The drawing under review shows one solid part. Ordinate dimensions are in mm from its lowest x, y, z. Coordinates: 2 decimals unless noted, no trailing zeros. Loops run counter-clockwise (first coordinate to the right, second up) from the corner with the lowest first, then second, coordinate; pieces in that order, holes last. Notation, with made-up numbers: (27, 86.5) - (71, 86.5) arc R9 ccw to (71, 99.5) - close; hole circle Ø10 at (-8.75, 89.25). An arc over 180 degrees is marked (long way). Answer as a JSON object with one key per item and string values. Group by question number.
Item 1: Clearance check with flat-ended pins moving along their axes: pin 1 (1.5 mm diameter, centred on x = 20.5, y = 2, fed in from +Z); pin 2 (1.5 mm diameter, centred on x = 60, y = 1, fed in from +Z). State where each tip first meets the part, or that it passes through.
Item 2: To check wall thickness, follow line 1 (Z direction, x = 17.5, y = 1.8); line 2 (X direction, y = 2.55, z = 16) (1 decimal); line 3 (X direction, y = 1.5, z = 35.5). State the ranges of each line that lie inside material, in increasing order.
Item 3: We need section B-B (x = 53.5). Give the boundary of the cut face in (y, z), then the cut area to 3 significant figures.
Item 4: We need section C-C (z = 7). Give the boundary of the cut face in (x, y).
Item 5: We need section A-A (z = 18). Give the boundary of the cut face in (x, y).
Item 6: We need section D-D (y = 1.2). Give the boundary of the cut face in (x, z).
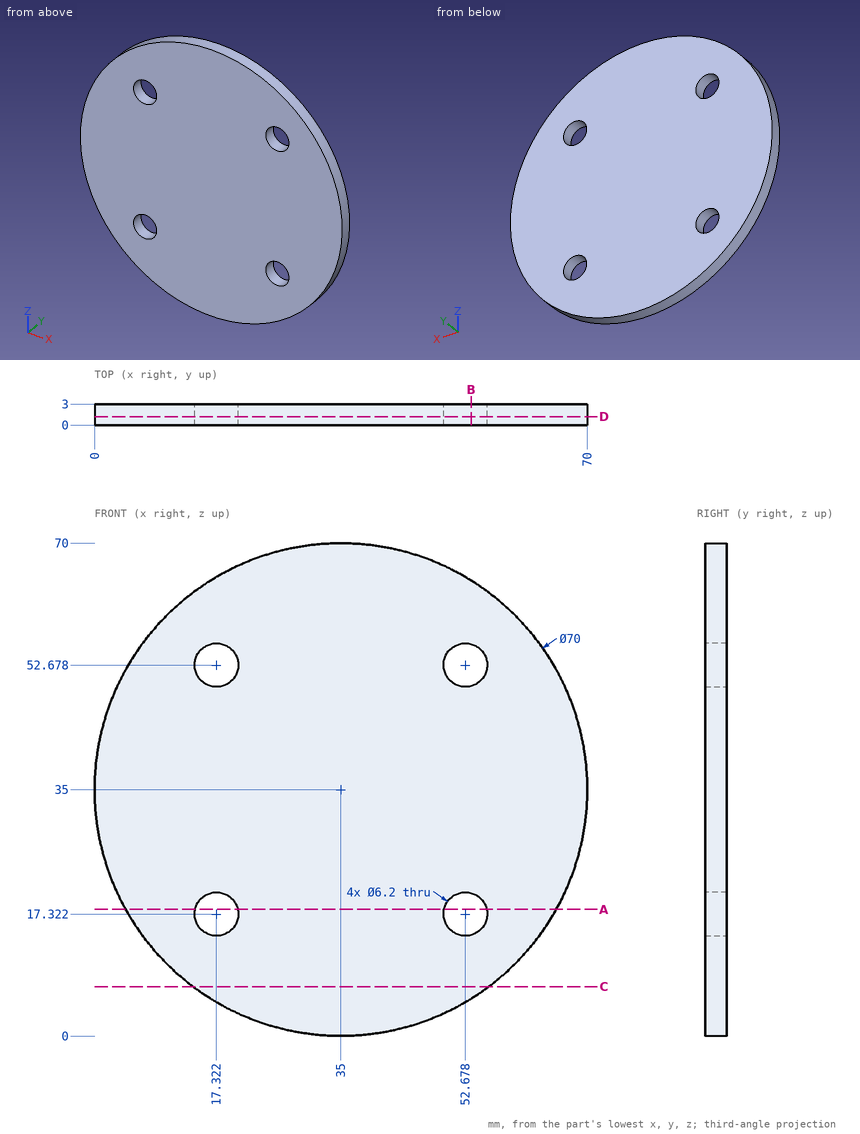
Check sheet entries:
{
 "1": {"pin 1": "stops at z = 67.19", "pin 2": "stops at z = 60.24"},
 "2": {"line 1": "z = 4.69 to 14.23, 20.42 to 49.58, 55.77 to 65.31", "line 2": "x = 5.6 to 14.5, 20.1 to 49.9, 55.5 to 64.4", "line 3": "x = 0 to 70"},
 "3": {"outline": "(0, 5.29) - (3, 5.29) - (3, 14.33) - (0, 14.33) - close; (0, 20.31) - (3, 20.31) - (3, 49.69) - (0, 49.69) - close; (0, 55.67) - (3, 55.67) - (3, 64.71) - (0, 64.71) - close", "area": "142 mm2"},
 "4": {"outline": "(14, 0) - (56, 0) - (56, 3) - (14, 3) - close"},
 "5": {"outline": "(4.41, 0) - (14.3, 0) - (14.3, 3) - (4.41, 3) - close; (20.35, 0) - (49.65, 0) - (49.65, 3) - (20.35, 3) - close; (55.7, 0) - (65.59, 0) - (65.59, 3) - (55.7, 3) - close"},
 "6": {"outline": "circle Ø70 at (35, 35); hole circle Ø6.2 at (17.32, 17.32); hole circle Ø6.2 at (17.32, 52.68); hole circle Ø6.2 at (52.68, 17.32); hole circle Ø6.2 at (52.68, 52.68)"}
}
